Autodesk Inventor part; units mm, degrees
ref_plane "YZ Plane" through (0, 0, 0) normal (1, 0, 0) x (0, 1, 0)
ref_plane "XZ Plane" through (0, 0, 0) normal (0, 1, 0) x (-1, 0, 0)
ref_plane "XY Plane" through (0, 0, 0) normal (0, 0, 1) x (1, 0, 0)
sketch "Sketch1" plane through (0, 0, 0) normal (0, 0, 1) x (1, 0, 0)
  line L0 (-200, 10) -> (200, 10)
  line L1 (200, 10) -> (200, -10)
  line L2 (200, -10) -> (-200, -10)
  line L3 (-200, -10) -> (-200, 10)
  circle A0 centre (-133.3333, 0) radius 2.15
  circle A1 centre (-66.6667, 0) radius 2.15
  circle A2 centre (0, 0) radius 2.15
  circle A3 centre (66.6667, 0) radius 2.15
  circle A4 centre (133.3333, 0) radius 2.15
  line L4 (-10, 10) -> (10, 10)
  line L5 (10, 10) -> (10, 30)
  line L6 (10, 30) -> (-10, 30)
  line L7 (-10, 30) -> (-10, 10)
  line L8 (-200, -10) -> (-201, -10)
  line L9 (-201, -10) -> (-201, 10)
  line L10 (-201, 10) -> (-200, 10)
  line L11 (-200, 10) -> (-200, -10)
  line L12 (200, -10) -> (201, -10)
  line L13 (201, -10) -> (201, 10)
  line L14 (201, 10) -> (200, 10)
  line L15 (200, 10) -> (200, -10)
  point P0 (0, 0)
  point P1 (0, 10)
  point P2 (200, 0)
  point P3 (-200, 0)
  point P4 (0, 30)
  dimension "d0" = 400
  dimension "d1" = 20
  dimension "d2" = 4.3
  dimension "d3" = 66.6667
  dimension "d6" = 66.6667
  dimension "d21" = 20
  dimension "d22" = 20
  dimension "d45" = 1
  dimension "d46" = 1
extrude "Extrusion1" add sketch "Sketch1" along normal blind 5
fillet "Fillet1" radius 10 4 edges at (10, 10, 2.5) (10, 30, 2.5) (-10, 10, 2.5) (-10, 30, 2.5)
extrude "Extrusion2" add sketch "Sketch1" along normal blind 3.2 contours A0 | A1 | A2 | A3 | A4
sketch "Sketch3" plane through (-190, 10, 0) normal (0, 1, 0) x (1, 0, 0)
  line L0 (190, 0) -> (190, -5)
  line L1 (390, -5) -> (210, -5)
  circle A0 centre (190, -2.5) radius 2
  line L2 (190.5, -4.5) -> (189.5, -4.5)
  line L3 (189.5, -4.5) -> (189.5, -0.5)
  line L4 (189.5, -0.5) -> (190.5, -0.5)
  line L5 (190.5, -0.5) -> (190.5, -4.5)
  point P0 (380, -5)
  point P1 (0, -5)
  point P2 (190, -4.5)
  point P3 (189.5, -2.5)
  point P4 (190.5, -0.5635)
  point P5 (190.5, -4.4365)
  dimension "d18" = 4
  dimension "d19" = 1
revolve "Revolution2" [suppressed]
sketch "Sketch4" plane through (0, 0, 0) normal (0, 0, -1) x (-1, 0, 0)
  arc A0 (10, 20) -> (-10, 20) centre (0, 20) ccw
  circle A1 centre (0, 20) radius 6
  line L0 (-6, 20) -> (6, 20)
  line L1 (6, 20) -> (6, 5)
  line L2 (6, 5) -> (-6, 5)
  line L3 (-6, 5) -> (-6, 13.2336)
  line L4 (-6, 20) -> (-4, 20)
  line L5 (-4, 20) -> (-4, 17.7057)
  line L6 (-6, 16.9596) -> (-6, 20)
  line L7 (0, 5) -> (0, 6)
  circle A2 centre (0, 11) radius 6
  arc A3 (-5, 15.4697) -> (-4, 17.7057) centre (-7, 17.7057) ccw
  arc A4 (-5, 15.4697) -> (-6, 13.2336) centre (-3, 13.2336) ccw
  line L8 (-6, 13.2336) -> (-6, 16.9596)
  line L9 (4, 20) -> (4, 17.7057)
  arc A5 (4, 17.7057) -> (5, 15.4697) centre (7, 17.7057) ccw
  arc A6 (6, 13.2336) -> (5, 15.4697) centre (3, 13.2336) ccw
  circle A7 centre (0, 20) radius 4
  point P0 (0, 0)
  point P1 (-4, 15)
  point P2 (6, 13.2336)
  point P3 (-6, 18.4798)
  point P4 (4.5061, 16.0383)
  point P5 (-4.5061, 16.0383)
  dimension "d36" = 8
  dimension "d38" = 2
  dimension "d25" = 15
  dimension "d27" = 2.8
  dimension "d28" = 5
  dimension "d30" = 3
  dimension "d39" = 12
extrude "Extrusion3" [suppressed]
extrude "Extrusion4" add sketch "Sketch4" against normal blind 1 contours L0 A7 A1 | L1 A6 A5 A1 | A1 A5 L9 L0 | L0 L5 A3 A1 | A1 A3 A4 L8 L6
ref_plane "Work Plane1" through (-4, 17.7057, 0) normal (0, -1, 0) x (1, 0, 0)
sketch "Sketch5" plane through (-4, 17.7057, 0) normal (0, -1, 0) x (1, 0, 0)
  line L0 (8, 1) -> (10, 3)
  line L1 (8, 1) -> (10.8284, 1) construction
  line L2 (10, 3) -> (10, 1)
  line L3 (10, 1) -> (8, 1)
  point P0 (4, 0)
  dimension "d40" = 45
sketch "Sketch6" plane through (0, 0, 0) normal (0, 0, -1) x (-1, 0, 0)
  line L0 (-4, 17.7057) -> (-4, 20)
  arc A0 (4, 20) -> (-4, 20) centre (0, 20) ccw
  line L1 (4, 20) -> (4, 17.7057)
  point P0 (0, 0)
sweep "Sweep1" [suppressed]
fillet "Fillet2" [suppressed]
fillet "Fillet3" radius 3 5 edges at (-10, 20, 0) (10, 20, 0) (7.0712, 27.0712, 0) (201, 0, 0) (-201, 0, 0)
sketch "Sketch7" plane through (0, 0, 5) normal (0, 0, 1) x (1, 0, 0)
  line L0 (-20, 10) -> (-201, 10)
  line L1 (-201, 10) -> (-200, 10)
  line L2 (-200, 10) -> (-200, 0)
  line L3 (-200, 0) -> (-201, 0)
  line L4 (-201, 0) -> (-201, 10)
  line L5 (-200, 10) -> (-190, 10)
  line L6 (-190, 10) -> (-190, 9)
  line L7 (-190, 9) -> (-200, 9)
  line L8 (-200, 9) -> (-200, 10)
  line L9 (0, 0) -> (0, 1.5374)
  line L10 (20, 10) -> (201, 10)
  line L11 (201, 10) -> (200, 10)
  line L12 (200, 10) -> (200, 0)
  line L13 (200, 0) -> (201, 0)
  line L14 (201, 0) -> (201, 10)
  line L15 (200, 10) -> (190, 10)
  line L16 (190, 10) -> (190, 9)
  line L17 (190, 9) -> (200, 9)
  line L18 (200, 9) -> (200, 10)
  line L19 (-200, 0) -> (-199.6, 0)
  line L20 (-199.6, 0) -> (-199.6, 9)
  line L21 (-199.6, 9) -> (-200, 9)
  line L22 (-200, 9) -> (-200, 0)
  line L23 (-190, 9) -> (-200, 9)
  line L24 (-200, 9) -> (-200, 8.6)
  line L25 (-200, 8.6) -> (-190, 8.6)
  line L26 (-190, 8.6) -> (-190, 9)
  line L27 (190, 9) -> (200, 9)
  line L28 (200, 9) -> (200, 8.6)
  line L29 (200, 8.6) -> (190, 8.6)
  line L30 (190, 8.6) -> (190, 9)
  line L31 (200, 0) -> (199.6, 0)
  line L32 (199.6, 0) -> (199.6, 8.6)
  line L33 (199.6, 8.6) -> (200, 8.6)
  line L34 (200, 8.6) -> (200, 0)
  point P0 (-199.6, 8.6)
  dimension "d47" = 1
  dimension "d48" = 10
  dimension "d49" = 10
  dimension "d50" = 1
  dimension "d53" = 0.4
  dimension "d54" = 0.4
  dimension "d55" = 0.4
  dimension "d56" = 0.4
extrude "Extrusion5" cut sketch "Sketch7" against normal blind 1
equation "\"d0\" = dolzina_drzala"
equation "\"d1\" = sirina_drzala"
equation "\"d2\" = fi_magneta + 2 * toleranca"
equation "\"d6\" = d3"
equation "\"d11\" = debelina_drzala"
equation "\"d14\" = -globina_luknje + debelina_drzala - toleranca"
equation "\"d39\" = d36 + 2 * d38"
equation "\"fi_magneta\" = 3.7"
equation "\"toleranca\" = 0.3"
equation "\"dolzina_drzala\" = 400"
equation "\"sirina_drzala\" = 20"
equation "\"debelina_drzala\" = 5"
equation "\"globina_luknje\" = 1.5"
properties part number "drzalo_za_poster_40x60_top"
Model file for the job. Use its own axes, mm. Give positions to 0.01 mm unless a question says otherwise; leave off trailing zeros. Order: outer loops, then holes, each group sorted by start corner. A loop starts at its lowest first (then second) coordinate and runs counter-clockwise, first axis right, second up. Notation, with made-up numbers: (76.25, -26) - (117.25, -26) arc R17 ccw to (117.25, -13) - close; hole circle Ø4 at (-11.5, 56.25). An arc over 180 degrees is marked (long way). Write item = value, one per line. Start each with the question number.
1. Probe line 1 along X through (y, z) = (0.5, 4.4); line 2 along Y through (x, z) = (143, 2.6); line 3 along X through (y, z) = (1, 4.45). List the from-to ranges inside material, lowest first.
2. Drop flat-ended pins along their axis: P1, Ø0.8, axis at x = -197, z = 4.5, coming from the +Y side; P2, Ø0.8, axis at y = 3.5, z = 4.5, coming from the -X side; P3, Ø2, axis at x = 133.5, y = 0.5, coming from the +Z side; P4, Ø1, axis at x = 137.5, y = 11, coming from the -Z side. Give the stop position or say it passes through.
3. Cut at B-B, the plane x = -38.5. List the corners of the cut face in (y, z), and give its area (3 significant figures).
Taken from the geometry:
q1.line_1 = -199.6 to -135.42, -131.24 to -68.76, -64.58 to -2.09, 2.09 to 64.58, 68.76 to 131.24, 135.42 to 199.6
q1.line_2 = -10 to 9.97
q1.line_3 = -199.6 to -135.24, -131.43 to -68.57, -64.76 to -1.9, 1.9 to 64.76, 68.57 to 131.43, 135.24 to 199.6
q2.P1 = 8.6
q2.P2 = -199.6
q2.P3 = 3.2
q2.P4 = through
q3.outline = (-10, 0) - (7, 0) arc R3 ccw to (10, 3) - (10, 5) - (-10, 5) - close
q3.area = 98.1 mm²
